from build123d import *

# Parameters (mm, degrees)
F0_W     = 31.75
F0_H     = 31.75
F0_W_2   = 25.4
F0_H_2   = 25.4
F1_DEPTH = 190.5
F3_DEPTH = 31.75
F5_DEPTH = 31.75


with BuildPart() as f1:
    # F0 (on Top) → F1 (new body, symmetric)
    with BuildSketch(Plane.XY):
        Rectangle(F0_W, F0_H)
        Rectangle(F0_W_2, F0_H_2, mode=Mode.SUBTRACT)
    extrude(amount=F1_DEPTH, both=True)

    # F2 (on face) → F3 (cut)
    with BuildSketch(Plane(origin=(-15.875, 0, 0), x_dir=(0, -1, 0), z_dir=(-1, 0, 0))):
        Polygon((15.875, 190.5), (-15.875, 190.5), (-15.875, 177.8), align=None)
    extrude(amount=-F3_DEPTH, mode=Mode.SUBTRACT)

    # F4 (on face) → F5 (cut)
    with BuildSketch(Plane(origin=(-15.875, 0, 0), x_dir=(0, -1, 0), z_dir=(-1, 0, 0))):
        Polygon((-15.875, -190.5), (15.875, -190.5), (15.875, -177.8), align=None)
    extrude(amount=-F5_DEPTH, mode=Mode.SUBTRACT)


solid = f1.part
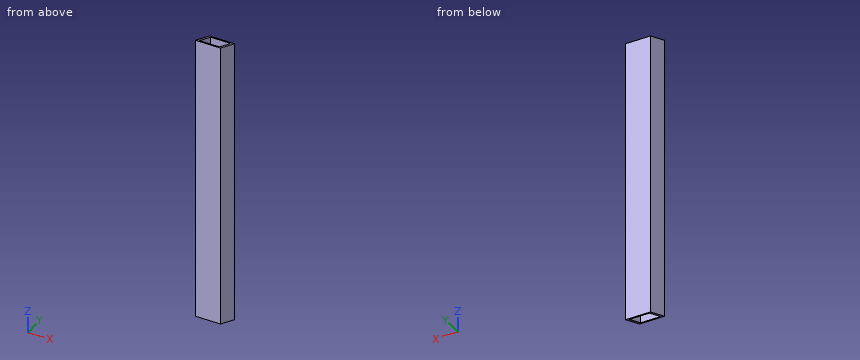
CAD build for the part. Positions are in the model's coordinates, mm. Round coordinates to 2 decimals unless told otherwise and drop trailing zeros. Loops run counter-clockwise (first coordinate to the right, second up) from the corner with the lowest first, then second, coordinate; pieces in that order, holes last.
(1) Cut at B-B (z = 35). Give the cut face in (x, y) (3 decimals), plus the area to 3 significant figures.
(2) Cut at A-A (x = 7). Give the cut face in (y, z) (3 decimals).
(3) Wall check: line 1 along X through (y, z) = (0.5, -80.5) (3 decimals); line 2 along Z through (x, y) = (13, -8.5). Give the ranges that are in metal, low to high.
(4) Cut at C-C (y = 9.5). Give the cut face in (x, z) (3 decimals).
Findings below:
1. outline: (-15.875, -15.875) - (15.875, -15.875) - (15.875, 15.875) - (-15.875, 15.875) - close; hole (-12.7, -12.7) - (12.7, -12.7) - (12.7, 12.7) - (-12.7, 12.7) - close
1. area: 363 mm2
2. outline: (-15.875, -177.8) - (-12.7, -179.07) - (-12.7, 189.23) - (-15.875, 190.5) - close; (12.7, -189.23) - (15.875, -190.5) - (15.875, 177.8) - (12.7, 179.07) - close
3. line 1: x = -15.875 to -12.7, 12.7 to 15.875
3. line 2: z = -180.75 to 187.55
4. outline: (-15.875, -187.95) - (-12.7, -187.95) - (-12.7, 180.35) - (-15.875, 180.35) - close; (12.7, -187.95) - (15.875, -187.95) - (15.875, 180.35) - (12.7, 180.35) - close
